The model under review builds one solid part; all positions refer to its coordinate system, in mm. Face numbers are marked on the shaded views. A direction names the side the tool comes from. Coordinates: 2 decimals unless noted, no trailing zeros. Write each loop counter-clockwise with the first axis right and the second up, starting at its lowest first coordinate (ties: lowest second). Pieces come first, ordered by that corner, then holes. Notation, with made-up numbers: (50, 74) - (109, 74) arc R29 ccw to (109, 107) - close; hole circle Ø3 at (47.25, -9). An arc over 180 degrees is marked (long way). Put each result on its own line as item: value. Start each with the question number.
Item 1: Consider section D-D on x = -14.5. Give the boundary of the cut face in (y, z).
Item 2: Machinability: for the marked faces 1, 2, 3, 4 and 5, which of the approach directions +Z, -Z, +X, -X, +Y, -Y give a long, thin tool a straight path to every point of the face, cutting with its end or side? Answer none if there is none.
Item 3: Consider section C-C on x = -8.5. Give the boundary of the cut face in (y, z).
Item 4: For pin 1 (3 mm diameter, centred on y = 7, z = 9, fed in from +X); pin 2 (12 mm diameter, centred on y = -0.5, z = 21, fed in from -X); pin 3 (5 mm diameter, centred on x = 12, y = -1.5, fed in from -Z), all flat-tipped, find the tip position at first contact; note any pin that passes through.
Item 5: To check wall thickness, follow L1, parallel to X at y = 9.5, z = 4; L2, parallel to X at y = -10, z = -27; L3, parallel to Y at x = 4.5, z = -22. State the ranges of each line that lie inside material, in increasing order. Write a range as [from, to].
Item 6: Consider section B-B on z = 23.5. Give the boundary of the cut face in (x, y), then the cut area to 3 significant figures.
Item 7: Mouldability with a two-part tool opening along X and no side actions: class the marked faces 6, 7 and 8 as pulls with the +X half, pulls with the -X half, needs draft (parallel to the pull), parting line crosses it, or undercut.
Item 8: Consider section A-A on y = -9.75. Give the boundary of the cut face in (x, z), then the cut area to 3 significant figures.
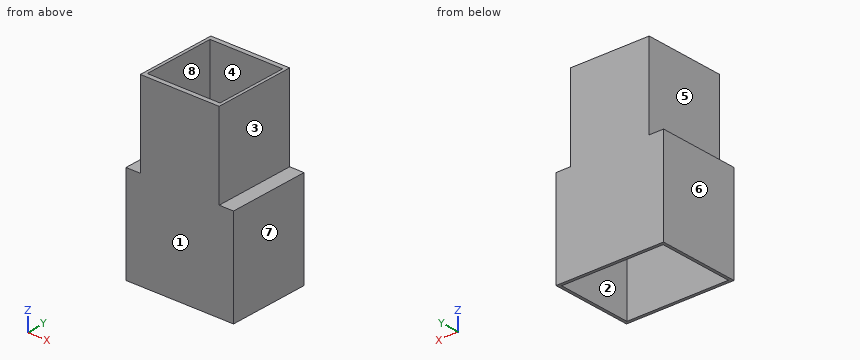
```python
from build123d import *

# Parameters (mm, degrees)
SKETCH_W      = 26
SKETCH_H      = 27
SKETCH_W_2    = 24
SKETCH_H_2    = 24
PAD_DEPTH     = 30
SKETCH001_W   = 35.5
SKETCH001_H   = 27
SKETCH001_W_2 = 33.5
SKETCH001_H_2 = 25
PAD001_DEPTH  = 30
SKETCH002_W   = 35.5
SKETCH002_H   = 27
SKETCH002_W_2 = 24
SKETCH002_H_2 = 24
PAD002_DEPTH  = 2


with BuildPart() as part:
    # Sketch → Pad (new body)
    with BuildSketch(Plane.XY):
        Rectangle(SKETCH_W, SKETCH_H)
        Rectangle(SKETCH_W_2, SKETCH_H_2, mode=Mode.SUBTRACT)
    extrude(amount=PAD_DEPTH)

    # Sketch001 → Pad001 (join)
    with BuildSketch(Plane.XY):
        Rectangle(SKETCH001_W, SKETCH001_H)
        Rectangle(SKETCH001_W_2, SKETCH001_H_2, mode=Mode.SUBTRACT)
    extrude(amount=-PAD001_DEPTH)

    # Sketch002 → Pad002 (join)
    with BuildSketch(Plane.XY):
        Rectangle(SKETCH002_W, SKETCH002_H)
        Rectangle(SKETCH002_W_2, SKETCH002_H_2, mode=Mode.SUBTRACT)
    extrude(amount=PAD002_DEPTH)


solid = part.part
```
Report:
1. outline: (-13.5, -30) - (-12.5, -30) - (-12.5, 0) - (12.5, 0) - (12.5, -30) - (13.5, -30) - (13.5, 2) - (-13.5, 2) - close
2. face 1: +Z, -Z, +X, -X, -Y
2. face 2: -Z
2. face 3: +Z, +X, +Y, -Y
2. face 4: +Z, -Z
2. face 5: +Z, -X, +Y, -Y
3. outline: (-13.5, -30) - (-12.5, -30) - (-12.5, 0) - (-12, 0) - (-12, 30) - (-13.5, 30) - close; (12, 0) - (12.5, 0) - (12.5, -30) - (13.5, -30) - (13.5, 30) - (12, 30) - close
4. pin 1: x = 13
4. pin 2: x = -13
4. pin 3: z = 0
5. L1: [-13, -12], [12, 13]
5. L2: [-17.75, -16.75], [16.75, 17.75]
5. L3: [-13.5, -12.5], [12.5, 13.5]
6. outline: (-13, -13.5) - (13, -13.5) - (13, 13.5) - (-13, 13.5) - close; hole (-12, -12) - (12, -12) - (12, 12) - (-12, 12) - close
6. area: 126 mm²
7. face 6: pulls with the -X half
7. face 7: pulls with the +X half
7. face 8: undercut
8. outline: (-17.75, -30) - (-16.75, -30) - (-16.75, 0) - (-12, 0) - (-12, 30) - (-13, 30) - (-13, 2) - (-17.75, 2) - close; (12, 0) - (16.75, 0) - (16.75, -30) - (17.75, -30) - (17.75, 2) - (13, 2) - (13, 30) - (12, 30) - close
8. area: 139 mm²
